The model under review builds one solid part; all positions refer to its coordinate system, in mm. A direction names the side the tool comes from. Coordinates: 2 decimals unless noted, no trailing zeros. Loops run counter-clockwise (first coordinate to the right, second up) from the corner with the lowest first, then second, coordinate; pieces in that order, holes last. Notation, with made-up numbers: (78, 17) - (115, 17) arc R26 ccw to (115, 34) - close; hole circle Ø7 at (10, -18). An arc over 180 degrees is marked (long way). One line per item, written item: value. Start each with the question number.
1. Insertion check: P1, Ø2.5, axis at x = 13.24, z = 4, coming from the +Y side; P2, Ø3, axis at x = -14, z = 5.5, coming from the +Y side; P3, Ø2, axis at x = 12.5, z = 4, coming from the +Y side; P4, Ø4.5, axis at y = 17, z = 4, coming from the -X side. Each pin has a flat end and moves straight along its axis. Give the tip position at first contact, or say it passes through.
2. We need section C-C, the plane y = 17. Give the boundary of the cut face in (x, z).
3. For faces 1 (the face through (8.521, 19.763, 4.881)), 2 (the face through (-16, 10, 6)), 3 (the face through (-8.37, 14.07, 3.35)), list the 3-axis set-ups (+Z, -Z, +X, -X, +Y, -Y) from which the entire face can be reached by the end or side of a thin tool; tool diameter is ignored.
4. To check wall thickness, follow line 1 (X direction, y = 5.25, z = 4.75); line 2 (X direction, y = 9.2, z = 4); line 3 (Y direction, x = -3, z = 3). State the ranges of each line that lie inside material, in increasing order.
5. We need section A-A, the plane y = 11. Give the boundary of the cut face in (x, z), then the cut area to 3 significant figures.
6. Mouldability with a two-part tool opening along Y and no side actions: class faces 4 (the face through (0, 6, 0)), 5 (the face through (7, 19, 5)), 6 (the face through (-6.7, 15.7, 5.3)), 7 (the face through (0, 0, 4)) as +Y half, -Y half, draft (parallel to the pull), parting line (faces both ways), or undercut.
7. We need section B-B, the plane x = 14.5. Give the boundary of the cut face in (y, z).
8. We need section D-D, the plane x = 9. Give the boundary of the cut face in (y, z).
from build123d import *

# Parameters (mm, degrees)
EXTRUDE_1_DEPTH     = 8
CUT_EXTRUDE_1_DEPTH = 9
SKETCH_3_R          = 1.65
CUT_EXTRUDE_2_DEPTH = 28
SKETCH_4_R          = 3
CUT_EXTRUDE_3_DEPTH = 3.3
CUT_EXTRUDE_4_DEPTH = 3
SKETCH_6_R          = 1.65
CUT_EXTRUDE_5_DEPTH = 11
SKETCH_7_R          = 3
CUT_EXTRUDE_6_DEPTH = 3.3


with BuildPart() as part:
    # 草图1 → 凸台-拉伸1 (new body)
    with BuildSketch(Plane.XY):
        Polygon((-10, 22), (10, 22), (10, 10), (17, 10), (17, 0), (-17, 0), (-17, 10), (-10, 10), align=None)
    extrude(amount=EXTRUDE_1_DEPTH)

    # 草图2 → 切除-拉伸1 (cut, through all)
    with BuildSketch(Plane.XY.offset(8)):
        with BuildLine():
            Line((-1, 22), (1, 22))
            Line((1, 22), (1, 14.872983346))
            ThreePointArc((1, 14.872983346), (0, 7), (-1, 14.872983346))
            Line((-1, 14.872983346), (-1, 22))
        make_face()
    extrude(amount=-CUT_EXTRUDE_1_DEPTH, mode=Mode.SUBTRACT)

    # 草图3 → 切除-拉伸2 (cut, through all)
    with BuildSketch(Plane.ZY.offset(10)):
        with Locations((4, 17)):
            Circle(SKETCH_3_R)
    extrude(amount=-CUT_EXTRUDE_2_DEPTH, mode=Mode.SUBTRACT)

    # 草图4 → 切除-拉伸3 (cut)
    with BuildSketch(Plane.ZY.offset(10)):
        with Locations((4, 17)):
            Circle(SKETCH_4_R)
    extrude(amount=-CUT_EXTRUDE_3_DEPTH, mode=Mode.SUBTRACT)

    # 草图5 → 切除-拉伸4 (cut)
    with BuildSketch(Plane(origin=(10, 0, 0), x_dir=(0, 0, -1), z_dir=(1, 0, 0))):
        Polygon((-6.494110918, 19.234444912), (-7.182141516, 15.957259041), (-4.688030598, 13.72281413), (-1.505889082, 14.765555088), (-0.817858484, 18.042740959), (-3.311969402, 20.27718587), align=None)
    extrude(amount=-CUT_EXTRUDE_4_DEPTH, mode=Mode.SUBTRACT)

    # 草图6 → 切除-拉伸5 (cut, through all)
    with BuildSketch(Plane(origin=(0, 10, 0), x_dir=(1, 0, 0), z_dir=(0, 1, 0))):
        with Locations((-13.239613272, -4)):
            Circle(SKETCH_6_R)
        with Locations((13.239613272, -4)):
            Circle(SKETCH_6_R)
    extrude(amount=-CUT_EXTRUDE_5_DEPTH, mode=Mode.SUBTRACT)

    # 草图7 → 切除-拉伸6 (cut)
    with BuildSketch(Plane(origin=(0, 10, 0), x_dir=(1, 0, 0), z_dir=(0, 1, 0))):
        with Locations((13.239613272, -4)):
            Circle(SKETCH_7_R)
        with Locations((-13.239613272, -4)):
            Circle(SKETCH_7_R)
    extrude(amount=-CUT_EXTRUDE_6_DEPTH, mode=Mode.SUBTRACT)


solid = part.part
Findings below:
1. P1: through
1. P2: y = 10
1. P3: y = 6.7
1. P4: x = -6.7
2. outline: (-10, 0) - (-1, 0) - (-1, 2.35) - (-6.7, 2.35) - (-6.7, 1) - (-10, 1) - close; (-10, 7) - (-6.7, 7) - (-6.7, 5.65) - (-1, 5.65) - (-1, 8) - (-10, 8) - close; (1, 0) - (10, 0) - (10, 1.04) - (7, 1.04) - (7, 2.35) - (1, 2.35) - close; (1, 5.65) - (7, 5.65) - (7, 6.96) - (10, 6.96) - (10, 8) - (1, 8) - close
3. face 1: +X
3. face 2: +Z, -Z, -X, +Y
3. face 3: -X
4. line 1: -17 to -14.71, -11.77 to 11.77, 14.71 to 17
4. line 2: -17 to -16.24, -10.24 to -3.57, 3.57 to 10.24, 16.24 to 17
4. line 3: 0 to 8.35, 13.65 to 15.69, 18.31 to 22
5. outline: (-10, 0) - (-4, 0) - (-4, 8) - (-10, 8) - close; (4, 0) - (10, 0) - (10, 8) - (4, 8) - close
5. area: 96.0 mm2
6. face 4: draft
6. face 5: undercut
6. face 6: undercut
6. face 7: -Y half
7. outline: (0, 0) - (10, 0) - (10, 1.28) - (6.7, 1.28) - (6.7, 2.94) - (0, 2.94) - close; (0, 5.06) - (6.7, 5.06) - (6.7, 6.72) - (10, 6.72) - (10, 8) - (0, 8) - close
8. outline: (0, 0) - (22, 0) - (22, 8) - (0, 8) - close; hole (13.72, 4.69) - (14.77, 1.51) - (18.04, 0.82) - (20.28, 3.31) - (19.23, 6.49) - (15.96, 7.18) - close
